The model under review builds one solid part; all positions refer to its coordinate system, in mm. Give positions to 0.01 mm unless a question says otherwise; leave off trailing zeros. Order: outer loops, then holes, each group sorted by start corner. A loop starts at its lowest first (then second) coordinate and runs counter-clockwise, first axis right, second up. Notation, with made-up numbers: (5, -38) - (20, -38) arc R26 cw to (20, -3) - close; hole circle Ø5 at (74, 76.5). An arc over 180 degrees is marked (long way). Write item = value, one per line. Start each with the question number.
1. We need section B-B, the plane z = -188. Give the boundary of the cut face in (x, y), and give its area (3 significant figures).
2. We need section C-C, the plane x = 163.5. Give the boundary of the cut face in (y, z), and give its area (3 significant figures).
3. For P1, Ø5, axis at x = 177.82, z = 36.16, coming from the +Y side, flat-tipped, find the tip position at first contact; note if it passes through.
4. We need section A-A, the plane y = 1.9. State how many separate pieces and enclosed holes the cut face has, and give its area (3 significant figures).
5. Wall thickness on probe 1 along Z at (x, y) = (0, 2.5); probe 2 along X at (y, z) = (0.75, 73); probe 3 along X at (y, z) = (1.6, -97.5): over which ranges is each line inside the solid? List them lowest first.
from build123d import *

# Parameters (mm, degrees)
BOSS_EXTRUDE2_DEPTH             = 3.12
CUT_EXTRUDE2_DEPTH              = 4.12
CUT_EXTRUDE3_DEPTH              = 4.12
F_1_4_0_25_DIAMETER_HOLE1_D     = 6.35
F_1_4_0_25_DIAMETER_HOLE1_DEPTH = 3.12
CUT_EXTRUDE4_REACH              = 5.12
SKETCH22_W                      = 62.565541267
SKETCH22_H                      = 30.394221155
F_6_0MM_DOWEL_HOLE2_D           = 6
F_6_0MM_DOWEL_HOLE2_DEPTH       = 3.12
F_6_0MM_DOWEL_HOLE1_D           = 6
F_6_0MM_DOWEL_HOLE1_DEPTH       = 3.12
F_6_0MM_DOWEL_HOLE3_D           = 6
F_6_0MM_DOWEL_HOLE3_DEPTH       = 3.12


with BuildPart() as part:
    # Sketch14 → Boss-Extrude2 (new body)
    with BuildSketch(Plane(origin=(0, 0, 0), x_dir=(1, 0, 0), z_dir=(0, 1, 0))):
        Polygon((224, 92.783837972), (92.783837972, 224), (-92.783837972, 224), (-224, 92.783837972), (-224, -92.783837972), (-92.783837972, -224), (92.783837972, -224), (224, -92.783837972), align=None)
    extrude(amount=BOSS_EXTRUDE2_DEPTH)

    # Sketch17 → Cut-Extrude2 (cut)
    with BuildSketch(Plane.XZ):
        Polygon((191.5, 125.283837972), (191.5, -125.741978826), (224, -92.783837972), (224, 92.783837972), align=None)
    extrude(amount=-CUT_EXTRUDE2_DEPTH, mode=Mode.SUBTRACT)

    # Sketch18 → Cut-Extrude3 (cut)
    with BuildSketch(Plane.XZ):
        Polygon((-191.5, 125.283837972), (-224, 92.783837972), (-224, -92.783837972), (-191.5, -125.283837972), align=None)
    extrude(amount=-CUT_EXTRUDE3_DEPTH, mode=Mode.SUBTRACT)

    # 1/4 (0.25) Diameter Hole1
    with Locations(Plane(origin=(0, 3.12, 0), x_dir=(1, 0, 0), z_dir=(0, 1, 0))):
        with Locations((67.963501684, -191.608983424), (-67.926498316, -191.608983424), (-129.064298316, -106.988883424), (-126.194098316, -70.895483424), (-126.194098316, -0.918483424), (-126.194098316, 69.058516576), (-14.103898316, 99.259116576), (108.730501684, 92.299516576), (126.231101684, 69.058516576), (126.231101684, -0.918483424), (129.101301684, -106.988883424), (126.231101684, -70.895483424), (0.018501684, -58.195483424)):
            Hole(F_1_4_0_25_DIAMETER_HOLE1_D / 2, depth=F_1_4_0_25_DIAMETER_HOLE1_DEPTH)

    # Sketch22 → Cut-Extrude4 (cut, up to next)
    with BuildSketch(Plane(origin=(0, 3.12, 0), x_dir=(1, 0, 0), z_dir=(0, 1, 0)), mode=Mode.PRIVATE) as cut_extrude4_sk1:
        with Locations((-0.116925735, -37.67927099)):
            Rectangle(SKETCH22_W, SKETCH22_H)
    cut_extrude4_tool1 = extrude(cut_extrude4_sk1.sketch, amount=-CUT_EXTRUDE4_REACH, mode=Mode.PRIVATE) & part.part
    add(cut_extrude4_tool1.solids().sort_by_distance((-0.116926, 3.12, 37.679271))[0], mode=Mode.SUBTRACT)

    # Ø6.0mm Dowel Hole2
    with Locations(Plane(origin=(0, 3.12, 0), x_dir=(1, 0, 0), z_dir=(0, 1, 0))):
        with Locations((-177.781498316, -36.158906441), (-177.781498316, -86.988906441), (-145.741498316, -36.158906441), (-145.741498316, -86.988906441), (145.778501684, -86.988906441), (177.818501684, -86.988906441), (177.818501684, -36.158906441), (145.778501684, -36.158906441)):
            Hole(F_6_0MM_DOWEL_HOLE2_D / 2, depth=F_6_0MM_DOWEL_HOLE2_DEPTH)

    # Ø6.0mm Dowel Hole1
    with Locations(Plane(origin=(0, 3.12, 0), x_dir=(1, 0, 0), z_dir=(0, 1, 0))):
        with Locations((-103.151498316, 84.807287956), (-124.001498316, 84.003641445)):
            Hole(F_6_0MM_DOWEL_HOLE1_D / 2, depth=F_6_0MM_DOWEL_HOLE1_DEPTH)

    # Ø6.0mm Dowel Hole3
    with Locations(Plane(origin=(0, 3.12, 0), x_dir=(1, 0, 0), z_dir=(0, 1, 0))):
        with Locations((-148.396200775, 75.127115617), (148.417336994, 75.150841329)):
            Hole(F_6_0MM_DOWEL_HOLE3_D / 2, depth=F_6_0MM_DOWEL_HOLE3_DEPTH)


solid = part.part
Model answer:
q1.outline = (-128.78, 0) - (128.78, 0) - (128.78, 3.12) - (-128.78, 3.12) - close
q1.area = 804 mm2
q2.outline = (0, -153.28) - (3.12, -153.28) - (3.12, 153.28) - (0, 153.28) - close
q2.area = 956 mm2
q3.P1 = through
q4.separate_pieces = 1
q4.enclosed_holes = 26
q4.area = 149,000 mm2
q5.probe_1 = -224 to 22.48, 52.88 to 55.02, 61.37 to 224
q5.probe_2 = -191.5 to -128.57, -123.82 to 123.85, 128.61 to 191.5
q5.probe_3 = -191.5 to -16.75, -11.46 to 191.5
